The figure shows three views and two pictorial views of one solid part (mm, origin at its lowest corner). Answer the questions. Coordinates: 2 decimals unless noted, no trailing zeros. Loops run counter-clockwise (first coordinate to the right, second up) from the corner with the lowest first, then second, coordinate; pieces in that order, holes last.
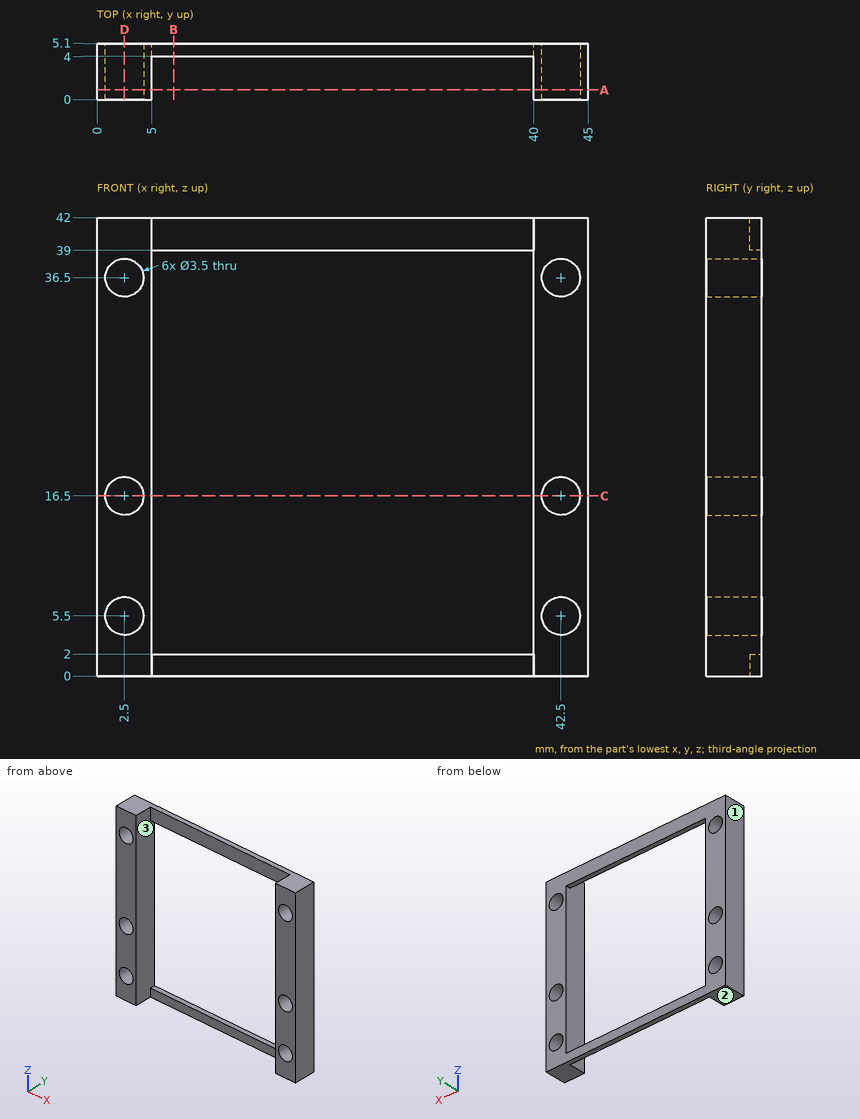
Q1. A cutting plane is placed at B-B (x = 7). Give the vertices of the cut face in (y, z), then the cut area to 3 significant figures.
Findings below:
outline: (4, 0) - (5.1, 0) - (5.1, 2) - (4, 2) - close; (4, 39) - (5.1, 39) - (5.1, 42) - (4, 42) - close
area: 5.50 mm2
Q2. A cutting plane is placed at A-A (y = 0.9). Give the vertices of the cut face in (x, z), then the cut area to 3 significant figures.
Findings below:
outline: (0, 0) - (5, 0) - (5, 42) - (0, 42) - close; (40, 0) - (45, 0) - (45, 42) - (40, 42) - close; hole circle Ø3.5 at (2.5, 5.5); hole circle Ø3.5 at (2.5, 16.5); hole circle Ø3.5 at (2.5, 36.5); hole circle Ø3.5 at (42.5, 5.5); hole circle Ø3.5 at (42.5, 16.5); hole circle Ø3.5 at (42.5, 36.5)
area: 362 mm2
Q3. A cutting plane is placed at C-C (z = 16.5). Give the vertices of the cut face in (x, y), then the cut area to 3 significant figures.
Findings below:
outline: (0, 0) - (0.75, 0) - (0.75, 5.1) - (0, 5.1) - close; (4.25, 0) - (5, 0) - (5, 5.1) - (4.25, 5.1) - close; (40, 0) - (40.75, 0) - (40.75, 5.1) - (40, 5.1) - close; (44.25, 0) - (45, 0) - (45, 5.1) - (44.25, 5.1) - close
area: 15.3 mm2
Q4. Determine the mould class of the marked faces 1, 2 and 3 for opening direction X: +X half, -X half, draft (parallel to the pull), parting line (faces both ways), or undercut.
Findings below:
face 1: -X half
face 2: draft
face 3: undercut
Q5. Straight lines are drawn through the part: probe 1 along Z at (x, y) = (2.5, 3.15); probe 2 along X at (y, z) = (3.1, 5.5); probe 3 along X at (y, z) = (0.8, 34). For each, find the intervals that lie inside material, in ascending order.
Findings below:
probe 1: z = 0 to 3.75, 7.25 to 14.75, 18.25 to 34.75, 38.25 to 42
probe 2: x = 0 to 0.75, 4.25 to 5, 40 to 40.75, 44.25 to 45
probe 3: x = 0 to 5, 40 to 45
Q6. A cutting plane is placed at D-D (x = 2.5). Give the vertices of the cut face in (y, z), then the cut area to 3 significant figures.
Findings below:
outline: (0, 0) - (5.1, 0) - (5.1, 3.75) - (0, 3.75) - close; (0, 7.25) - (5.1, 7.25) - (5.1, 14.75) - (0, 14.75) - close; (0, 18.25) - (5.1, 18.25) - (5.1, 34.75) - (0, 34.75) - close; (0, 38.25) - (5.1, 38.25) - (5.1, 42) - (0, 42) - close
area: 161 mm2
Q7. A flat-ended cylindrical pin translates along its axis: pin 1 Ø0.6 at (x, z) = (16.5, 1.5) entering from -Y. Find the tip coordinate at first contact, or state that the pin passes through.
Findings below:
pin 1: stops at y = 4
